```python
from build123d import *

# Parameters (mm, degrees)
SKETCH1_R           = 67.15
BOSS_EXTRUDE1_DEPTH = 5
SKETCH1_3_R         = 57.15
BOSS_EXTRUDE2_DEPTH = 2
SKETCH2_R           = 2.775
CUT_EXTRUDE1_DEPTH  = 2.89
CUT_EXTRUDE2_REACH  = 97.053
SKETCH3_R           = 1.6
FILLET1_R           = 5


with BuildPart() as part:
    # Sketch1 → Boss-Extrude1 (new body)
    with BuildSketch(Plane(origin=(0, 0, 0), x_dir=(1, 0, 0), z_dir=(0, 1, 0))):
        with Locations(Location((0, 0, 0), (0, 0, 270))):
            Circle(SKETCH1_R)
    extrude(amount=BOSS_EXTRUDE1_DEPTH)

    # Sketch1<3> → Boss-Extrude2 (add)
    with BuildSketch(Plane(origin=(0, 0, 0), x_dir=(1, 0, 0), z_dir=(0, 1, 0))):
        with Locations(Location((0, 0, 0), (0, 0, 270))):
            Circle(SKETCH1_3_R)
    extrude(amount=-BOSS_EXTRUDE2_DEPTH)

    # Sketch2 → Cut-Extrude1 (cut)
    with BuildSketch(Plane(origin=(0, 5, 0), x_dir=(1, 0, 0), z_dir=(0, 1, 0))):
        with Locations(Location((0, 0, 0), (0, 0, 270))):
            Circle(SKETCH2_R)
    extrude(amount=-CUT_EXTRUDE1_DEPTH, mode=Mode.SUBTRACT)

    # Sketch3 → Cut-Extrude2 (cut, up to next)
    with BuildSketch(Plane(origin=(0, 2.11, 0), x_dir=(1, 0, 0), z_dir=(0, 1, 0)), mode=Mode.PRIVATE) as cut_extrude2_sk1:
        with Locations(Location((0, 0, 0), (0, 0, 270))):
            Circle(SKETCH3_R)
    cut_extrude2_tool1 = extrude(cut_extrude2_sk1.sketch, amount=-CUT_EXTRUDE2_REACH, mode=Mode.PRIVATE) & part.part
    add(cut_extrude2_tool1.solids().sort_by_distance((0, 2.11, 0))[0], mode=Mode.SUBTRACT)

    # Fillet1
    fillet1_edges = [part.edges().sort_by_distance(p)[0] for p in [
        (0, 5, -67.15),
    ]]
    fillet(fillet1_edges, radius=FILLET1_R - 0.0001)  # a hair under: the kernel refuses the full size


solid = part.part
```
Input: part model. Units: mm. Frame: model coordinates. A direction names the side the tool comes from. Round coordinates to 2 decimals unless told otherwise and drop trailing zeros. Use one line per item in the form item = value. Start each with the question number.
Item 1: Material intervals for L1, parallel to Y at x = -40.5, z = -46.5; L2, parallel to X at y = 1.5, z = 28.5; L3, parallel to X at y = -1, z = -32, sorted ascending. Write a range as from..to.
Item 2: Set-up query: faces 1 (the face through (55, 0, 20)), 2 (the face through (2.34, 3.58, 1.49)), 3 (the face through (-12, -2, -1)). Return all of +Z, -Z, +X, -X, +Y, -Y with unobstructed straight access to the full face (end or side cutting, diameter ignored); none if empty.
Item 3: Contact query for a flat-ended pin moving along its axis: pin 1 Ø1.5 at (y, z) = (3.5, -10.5) entering from -X. Output: stop coordinate, or through.
Item 4: Mould query, pull axis X, two halves, no side actions, for faces 4 (the face through (-2, 2.11, 0)), 5 (the face through (2.513, -0.986, -57.095)), 6 (the face through (1, 5, 13)). Classes: pulls with the +X half, pulls with the -X half, needs draft (parallel to the pull), parting line crosses it, or undercut.
Ans:
q1.L1 = 0..5
q1.L2 = -60.55..60.55
q1.L3 = -47.35..47.35
q2.face_1 = -Y
q2.face_2 = +Y
q2.face_3 = +Z, -Z, +X, -X, -Y
q3.pin_1 = -65.5
q4.face_4 = undercut
q4.face_5 = parting line crosses it
q4.face_6 = needs draft
